Read the model definition and answer for the solid it produces. Units are mm, in the model's axes. Face numbers are marked on the shaded views. A direction names the side the tool comes from. Give positions to 0.01 mm unless a question says otherwise; leave off trailing zeros. Write each loop counter-clockwise with the first axis right and the second up, starting at its lowest first coordinate (ties: lowest second). Pieces come first, ordered by that corner, then holes. Notation, with made-up numbers: (-30.75, 81) - (14.25, 81) arc R25 ccw to (14.25, 101) - close; hole circle Ø9 at (58.5, 87). An arc over 180 degrees is marked (long way). Answer as a JSON object with one key per item and string values. Group by question number.
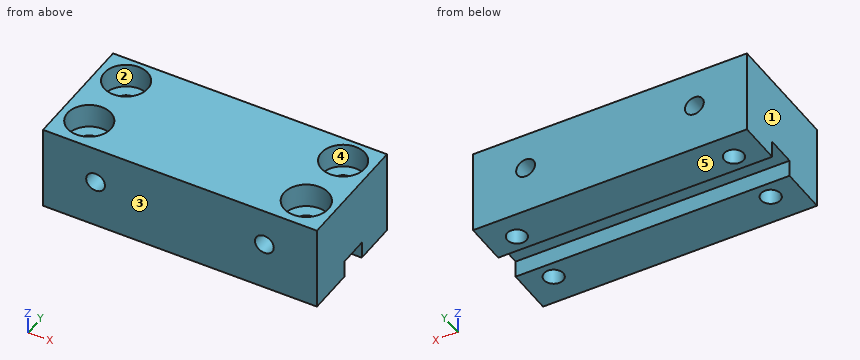
```python
from build123d import *

# Parameters (mm, degrees)
SKETCH1_W           = 72.136
SKETCH1_H           = 31.75
SKETCH1_R           = 5.715
SKETCH1_R_2         = 5.842
BOSS_EXTRUDE1_DEPTH = 22.352
SKETCH4_R           = 5.715
SKETCH4_R_2         = 2.54
SKETCH4_R_3         = 5.842
BOSS_EXTRUDE2_DEPTH = 16.002
SKETCH2_R           = 2.4765
CUT_EXTRUDE1_DEPTH  = 32.75
SKETCH5_W           = 4.445
SKETCH5_H           = 7.874
CUT_EXTRUDE2_DEPTH  = 73.136


with BuildPart() as part:
    # Sketch1 → Boss-Extrude1 (new body)
    with BuildSketch(Plane.XY):
        Rectangle(SKETCH1_W, SKETCH1_H)
        with Locations((-28.575, 8.875537672)):
            Circle(SKETCH1_R, mode=Mode.SUBTRACT)
        with Locations((28.575, 8.875537672)):
            Circle(SKETCH1_R, mode=Mode.SUBTRACT)
        with Locations((-28.575, -7.8002595)):
            Circle(SKETCH1_R, mode=Mode.SUBTRACT)
        with Locations((28.575, -7.8002595)):
            Circle(SKETCH1_R_2, mode=Mode.SUBTRACT)
    extrude(amount=BOSS_EXTRUDE1_DEPTH)

    # Sketch4 → Boss-Extrude2 (add)
    with BuildSketch(Plane.XY):
        with Locations((-28.575, 8.875537672)):
            Circle(SKETCH4_R)
        with Locations((-28.575, 8.875537672)):
            Circle(SKETCH4_R_2, mode=Mode.SUBTRACT)
        with Locations((-28.575, -7.8002595)):
            Circle(SKETCH4_R)
        with Locations((-28.575, -7.8002595)):
            Circle(SKETCH4_R_2, mode=Mode.SUBTRACT)
        with Locations((28.575, 8.875537672)):
            Circle(SKETCH4_R)
        with Locations((28.575, 8.875537672)):
            Circle(SKETCH4_R_2, mode=Mode.SUBTRACT)
        with Locations((28.575, -7.8002595)):
            Circle(SKETCH4_R_3)
        with Locations((28.575, -7.8002595)):
            Circle(SKETCH4_R_2, mode=Mode.SUBTRACT)
    extrude(amount=BOSS_EXTRUDE2_DEPTH)

    # Sketch2 → Cut-Extrude1 (cut, through all)
    with BuildSketch(Plane.XZ.offset(15.875)):
        with Locations((-22.225, 12.6365)):
            Circle(SKETCH2_R)
        with Locations((22.225, 12.6365)):
            Circle(SKETCH2_R)
    extrude(amount=-CUT_EXTRUDE1_DEPTH, mode=Mode.SUBTRACT)

    # Sketch5 → Cut-Extrude2 (cut, through all)
    with BuildSketch(Plane.ZY.offset(36.068)):
        with Locations((2.2225, 0.508)):
            Rectangle(SKETCH5_W, SKETCH5_H)
    extrude(amount=-CUT_EXTRUDE2_DEPTH, mode=Mode.SUBTRACT)


solid = part.part
```
1) For a pull along X with two mould halves and no side action, classify the marked faces 1, 2 and 3 as released by +X, released by -X, zero draft, split by the parting line, or undercut.
2) Find section D-D, the plane z = 8.75. Write down the section's boundary in (x, y) (3 decimals).
3) Find the intervals of material crossed by line 1 (X direction, y = 8.5, z = 20.25); line 2 (X direction, y = 5, z = 17.75); line 3 (Y direction, x = -20.5, z = 4.25) (3 decimals), in increasing order. Write a range as [from, to].
4) Find section B-B, the plane y = -6.5. Write down the section's boundary in (x, z) (1 decimal).
5) Find section C-C, the plane x = 29.5. Write down the section's boundary in (y, z) (3 decimals), and give its area (3 significant figures).
6) Which of the six approach directions +Z, -Z, +X, -X, +Y, -Y give full straight-line access (tool end or side, diameter ignored) to the marked faces 4 and 5?
7) Flat-ended cylindrical pins translate along their axes: pin 1 Ø4 at (x, y) = (-28.58, 8.88) entering from +Z; pin 2 Ø10.5 at (x, y) = (28.58, 8.88) entering from +Z. Find the tip coordinate at first contact, or state that the pin passes through.
8) Find section A-A, the plane z = 13.5. Write down the section's boundary in (x, y) (3 decimals), and give its area (3 significant figures).
Values follow:
{
 "1": {"face 1": "released by -X", "face 2": "undercut", "face 3": "zero draft"},
 "2": {"outline": "(-36.068, -15.875) - (36.068, -15.875) - (36.068, 15.875) - (-36.068, 15.875) - close; hole circle Ø5.08 at (-28.575, -7.8); hole circle Ø5.08 at (-28.575, 8.876); hole circle Ø5.08 at (28.575, -7.8); hole circle Ø5.08 at (28.575, 8.876)"},
 "3": {"line 1": "x = [-36.07, -34.28], [-22.87, 22.87], [34.28, 36.07]", "line 2": "x = [-36.07, -32.78], [-24.37, 24.37], [32.78, 36.07]", "line 3": "y = [-15.875, -3.429], [4.445, 15.875]"},
 "4": {"outline": "(-36.1, 0) - (-30.8, 0) - (-30.8, 16) - (-34.1, 16) - (-34.1, 22.4) - (-36.1, 22.4) - close; (-26.4, 0) - (26.4, 0) - (26.4, 16) - (22.9, 16) - (22.9, 22.4) - (-23, 22.4) - (-23, 16) - (-26.4, 16) - close; (30.8, 0) - (36.1, 0) - (36.1, 22.4) - (34.3, 22.4) - (34.3, 16) - (30.8, 16) - close; hole circle Ø5 at (-22.2, 12.6); hole circle Ø5 at (22.2, 12.6)"},
 "5": {"outline": "(-15.875, 0) - (-10.166, 0) - (-10.166, 16.002) - (-13.569, 16.002) - (-13.569, 22.352) - (-15.875, 22.352) - close; (-5.435, 0) - (-3.429, 0) - (-3.429, 4.445) - (4.445, 4.445) - (4.445, 0) - (6.51, 0) - (6.51, 16.002) - (3.236, 16.002) - (3.236, 22.352) - (-2.032, 22.352) - (-2.032, 16.002) - (-5.435, 16.002) - close; (11.241, 0) - (15.875, 0) - (15.875, 22.352) - (14.515, 22.352) - (14.515, 16.002) - (11.241, 16.002) - close", "area": "378 mm2"},
 "6": {"face 4": "+Z", "face 5": "-Z, +X, -X, +Y, -Y"},
 "7": {"pin 1": "passes through", "pin 2": "stops at z = 16"},
 "8": {"outline": "(-36.068, -15.875) - (-24.546, -15.875) - (-24.546, 15.875) - (-36.068, 15.875) - close; (-19.904, -15.875) - (19.904, -15.875) - (19.904, 15.875) - (-19.904, 15.875) - close; (24.546, -15.875) - (36.068, -15.875) - (36.068, 15.875) - (24.546, 15.875) - close; hole circle Ø5.08 at (-28.575, -7.8); hole circle Ø5.08 at (-28.575, 8.876); hole circle Ø5.08 at (28.575, -7.8); hole circle Ø5.08 at (28.575, 8.876)", "area": "1,910 mm2"}
}
